The model under review builds one solid part; all positions refer to its coordinate system, in mm. A direction names the side the tool comes from. Coordinates: 2 decimals unless noted, no trailing zeros. Write each loop counter-clockwise with the first axis right and the second up, starting at its lowest first coordinate (ties: lowest second). Pieces come first, ordered by that corner, then holes.
1) For P1, Ø3, axis at x = 0, z = 0, coming from the +Y side; P2, Ø1.5, axis at x = -3.5, y = 11.5, coming from the -Z side; P3, Ø1, axis at y = 12.5, z = 1, coming from the -X side, all flat-tipped, find the tip position at first contact; note any pin that passes through.
2) Add section B-B, the plane y = 17.25. State the section outline as (x, z) points, then the cut area to 3 significant figures.
3) For line 1 (Z direction, x = 1.25, y = 1.5); line 2 (X direction, y = 5.5, z = 0.75); line 3 (Y direction, x = -0.5, z = 0), list the stretches that pass through material, from the lowest coordinate up.
4) Add section D-D, the plane z = -3. State the section outline as (x, y) points, then the cut area to 3 significant figures.
5) Mouldability with a two-part tool opening along X and no side actions: class faces 4 (the cylindrical face through (-1, 16.96, -1.31)), 5 (the flat face through (-3.48, 9.86, -1.97)), 6 (the flat face through (3.448, 9.86, -2.028)) as released by +X, released by -X, zero draft, split by the parting line, or undercut.
6) Machinability: for faces 1 (the cylindrical face through (-1, 2.96, -1.31)), 2 (the flat face through (0, 14, 0)), 3 (the flat face through (3.48, 9.86, 1.97)), which of the approach directions +Z, -Z, +X, -X, +Y, -Y give a long, thin tool a straight path to every point of the face, cutting with its end or side? Answer none if there is none.
7) Add section C-C, the plane y = 12.25. State the section outline as (x, z) points, then the cut area to 3 significant figures.
8) Add section A-A, the plane x = 0. State the section outline as (y, z) points.
from build123d import *

# Parameters (mm, degrees)
EXTRUDE_1_DEPTH     = 20
SKETCH_2_R          = 1.65
CUT_EXTRUDE_1_DEPTH = 6
CUT_EXTRUDE_START   = -6
SKETCH_3_R          = 1.65
CUT_EXTRUDE_2_DEPTH = 6


with BuildPart() as part:
    # 草图1 → 凸台-拉伸1 (new body)
    with BuildSketch(Plane(origin=(0, 0, 0), x_dir=(1, 0, 0), z_dir=(0, 1, 0))):
        Polygon((4.618802154, 0), (2.309401077, -4), (-2.309401077, -4), (-4.618802154, 0), (-2.309401077, 4), (2.309401077, 4), align=None)
    extrude(amount=EXTRUDE_1_DEPTH)

    # 草图2 → 切除-拉伸1 (cut)
    with BuildSketch(Plane(origin=(0, 0, 0), x_dir=(1, 0, 0), z_dir=(0, 1, 0))):
        with Locations(Location((0, 0, 0), (0, 0, 270))):
            Circle(SKETCH_2_R)
    extrude(amount=CUT_EXTRUDE_1_DEPTH, mode=Mode.SUBTRACT)

    # 草图3 → 切除-拉伸2 (cut)
    with BuildSketch(Plane(origin=(0, 20, 0), x_dir=(1, 0, 0), z_dir=(0, 1, 0)).offset(CUT_EXTRUDE_START)):
        with Locations(Location((0, 0, 0), (0, 0, 270))):
            Circle(SKETCH_3_R)
    extrude(amount=CUT_EXTRUDE_2_DEPTH, mode=Mode.SUBTRACT)


solid = part.part
Geometry results:
1. P1: stops at y = 14
1. P2: stops at z = -3.24
1. P3: stops at x = -4.33
2. outline: (-4.62, 0) - (-2.31, -4) - (2.31, -4) - (4.62, 0) - (2.31, 4) - (-2.31, 4) - close; hole circle Ø3.3 at (0, 0)
2. area: 46.9 mm2
3. line 1: z = -4 to -1.08, 1.08 to 4
3. line 2: x = -4.19 to -1.47, 1.47 to 4.19
3. line 3: y = 6 to 14
4. outline: (-2.89, 0) - (2.89, 0) - (2.89, 20) - (-2.89, 20) - close
4. area: 115 mm2
5. face 4: undercut
5. face 5: released by -X
5. face 6: released by +X
6. face 1: -Y
6. face 2: +Y
6. face 3: +Z, +X, +Y, -Y
7. outline: (-4.62, 0) - (-2.31, -4) - (2.31, -4) - (4.62, 0) - (2.31, 4) - (-2.31, 4) - close
7. area: 55.4 mm2
8. outline: (0, -4) - (20, -4) - (20, -1.65) - (14, -1.65) - (14, 1.65) - (20, 1.65) - (20, 4) - (0, 4) - (0, 1.65) - (6, 1.65) - (6, -1.65) - (0, -1.65) - close
